from build123d import *

# Parameters (mm, degrees)
BOSS_EXTRUDE1_DEPTH = 20
CUT_EXTRUDE1_DEPTH  = 2.5
SKETCH4_R           = 2.25
CUT_EXTRUDE2_DEPTH  = 10
SKETCH5_W           = 12.8
SKETCH5_H           = 23.5
CUT_EXTRUDE3_DEPTH  = 16
SKETCH6_R           = 1
CUT_EXTRUDE4_DEPTH  = 6


with BuildPart() as part:
    # Sketch2 → Boss-Extrude1 (new body)
    with BuildSketch(Plane.XY):
        with BuildLine():
            Line((18.766775804, 101.178603266), (25.022367739, 1.571471021))
            ThreePointArc((25.022367739, 1.571471021), (0, -25.07166545), (-25.022367739, 1.571471021))
            Line((-25.022367739, 1.571471021), (-18.766775804, 101.178603266))
            ThreePointArc((-18.766775804, 101.178603266), (0, 118.803749087), (18.766775804, 101.178603266))
        make_face()
    extrude(amount=BOSS_EXTRUDE1_DEPTH)

    # Sketch3 → Cut-Extrude1 (cut)
    with BuildSketch(Plane.XY.offset(20)):
        with BuildLine():
            Line((-3, -10), (-3, -2.645751311))
            ThreePointArc((-3, -2.645751311), (-4, 0), (-3, 2.645751311))
            Line((-3, 2.645751311), (-3, 10))
            ThreePointArc((-3, 10), (0, 13), (3, 10))
            Line((3, 10), (3, 2.645751311))
            ThreePointArc((3, 2.645751311), (4, 0), (3, -2.645751311))
            Line((3, -2.645751311), (3, -10))
            ThreePointArc((3, -10), (0, -13), (-3, -10))
        make_face()
    extrude(amount=-CUT_EXTRUDE1_DEPTH, mode=Mode.SUBTRACT)

    # Sketch4 → Cut-Extrude2 (cut)
    with BuildSketch(Plane.XY.offset(17.5)):
        Circle(SKETCH4_R)
    extrude(amount=-CUT_EXTRUDE2_DEPTH, mode=Mode.SUBTRACT)

    # Sketch5 → Cut-Extrude3 (cut)
    with BuildSketch(Plane(origin=(0, 0, 0), x_dir=(-1, 0, 0), z_dir=(0, 0, -1))):
        with Locations((0, 94.25)):
            Rectangle(SKETCH5_W, SKETCH5_H)
    extrude(amount=-CUT_EXTRUDE3_DEPTH, mode=Mode.SUBTRACT)

    # Sketch6 → Cut-Extrude4 (cut)
    with BuildSketch(Plane(origin=(0, 0, 0), x_dir=(-1, 0, 0), z_dir=(0, 0, -1))):
        with Locations((0, 108.6)):
            Circle(SKETCH6_R)
        with Locations((0, 79.9)):
            Circle(SKETCH6_R)
    extrude(amount=-CUT_EXTRUDE4_DEPTH, mode=Mode.SUBTRACT)


solid = part.part
Work out the finished part from the listing and answer in its coordinate system (mm). A direction names the side the tool comes from. Give positions to 0.01 mm unless a question says otherwise; leave off trailing zeros. Loops run counter-clockwise (first coordinate to the right, second up) from the corner with the lowest first, then second, coordinate; pieces in that order, holes last. Notation, with made-up numbers: (23.25, 64.25) - (70.25, 64.25) arc R12 cw to (70.25, 82.25) - close; hole circle Ø6 at (28.25, 84). An arc over 180 degrees is marked (long way). Answer in a Markdown table with one row per item.
(1) Consider L1, parallel to Y at x = 0, z = 2.05; L2, parallel to X at y = 57, z = 5.5; L3, parallel to X at y = 79.9, z = 4. Determine where each line is inside the solid, lowest interval first. Write a range as [from, to].
Results list:
| item | result |
|---|---|
| L1 | y = [-25.07, 78.9], [80.9, 82.5], [106, 107.6], [109.6, 118.8] |
| L2 | x = [-21.54, 21.54] |
| L3 | x = [-20.1, -1], [1, 20.1] |
(2) For a pull along X with two mould halves and no side action, classify faces 1 (the face through (-4, 0, 19)), 2 (the face through (-21.94, 50.68, 9.86)), 3 (the face through (0, 48, 20)), 4 (the face through (21.85, 52.07, 9.86)) as pulls with the +X half, pulls with the -X half, needs draft (parallel to the pull), parting line crosses it, or undercut.
Results list:
| item | result |
|---|---|
| face 1 | undercut |
| face 2 | pulls with the -X half |
| face 3 | needs draft |
| face 4 | pulls with the +X half |
(3) A tool of negligible diameter and unlimited length cuts with its end or side. For faces 5 (the face through (0, 0, 7.5)), 6 (the face through (0, 82.5, 8)), 7 (the face through (0, 48, 0)), from which of +Z, -Z, +X, -X, +Y, -Y can it reach the whole face along a straight path? Write none if from no direction.
Results list:
| item | result |
|---|---|
| face 5 | +Z |
| face 6 | -Z |
| face 7 | -Z, +X, -X, +Y, -Y |
(4) Section C-C (x = -21) is taken. Give the vertices of the cut face in (y, z), and give its area (3 significant figures).
Results list:
| item | result |
|---|---|
| outline | (-13.7, 0) - (65.62, 0) - (65.62, 20) - (-13.7, 20) - close |
| area | 1,590 mm² |
(5) Section B-B (y = -6.5) is taken. Give the vertices of the cut face in (x, z), and give its area (3 significant figures).
Results list:
| item | result |
|---|---|
| outline | (-24.21, 0) - (24.21, 0) - (24.21, 20) - (3, 20) - (3, 17.5) - (-3, 17.5) - (-3, 20) - (-24.21, 20) - close |
| area | 954 mm² |
(6) Flat-ended cylindrical pins translate along their axes: pin 1 Ø2 at (y, z) = (6.5, 19.5) entering from -X; pin 2 Ø1 at (y, z) = (67, 8.5) entering from -X; pin 3 Ø10 at (y, z) = (-6, 5) entering from -X. Find the tip coordinate at first contact, or state that the pin passes through.
Results list:
| item | result |
|---|---|
| pin 1 | stops at x = -24.78 |
| pin 2 | stops at x = -20.94 |
| pin 3 | stops at x = -25.05 |
(7) Section A-A (z = 10.5) is taken. Give the vertices of the cut face in (x, y).
Results list:
| item | result |
|---|---|
| outline | (-25.02, 1.57) arc R25.07 ccw (long way) to (25.02, 1.57) - (18.77, 101.18) arc R18.8 ccw to (-18.77, 101.18) - close; hole (-6.4, 82.5) - (6.4, 82.5) - (6.4, 106) - (-6.4, 106) - close; hole circle Ø4.5 at (0, 0) |
(8) Section D-D (y = 54) is taken. Give the vertices of the cut face in (x, z), and give its area (3 significant figures).
Results list:
| item | result |
|---|---|
| outline | (-21.73, 0) - (21.73, 0) - (21.73, 20) - (-21.73, 20) - close |
| area | 869 mm² |
